Build history of the part. All positions in model axes, mm. A direction names the side the tool comes from. Round coordinates to 2 decimals unless told otherwise and drop trailing zeros. Write each loop counter-clockwise with the first axis right and the second up, starting at its lowest first coordinate (ties: lowest second). Pieces come first, ordered by that corner, then holes. Notation, with made-up numbers: (0, -38) - (15, -38) arc R28 ccw to (15, -8) - close; hole circle Ø11 at (22, -21.75). An arc over 180 degrees is marked (long way). Answer as a JSON object with one key per item and string values. Group by question number.
Item 1: Slice it at C-C, the plane z = 18. List the corners of the cut face in (x, y), then the cut area to 3 significant figures.
Item 2: Probe line 1 (Y direction, x = 7, z = 22.5); line 2 (Y direction, x = 2.5, z = -18.5); line 3 (X direction, y = 3.1, z = 18). List the from-to ranges inside material, lowest first. Write a range as from..to.
Item 3: Two-plate mould, pull along Z, no slides. Class faces 1 (the flat face through (15.586, 1.232, 1.42)), 2 (the flat face through (0, -66, -2.425)), 3 (the flat face through (0, -126, 0)): +Z half, -Z half, draft (parallel to the pull), parting line (faces both ways), or undercut.
Item 4: Slice it at A-A, the plane x = -18. List the corners of the cut face in (y, z).
Item 5: Which spindle directions (+Z, -Z, +X, -X, +Y, -Y) get a long thin tool onto all of the face, cutting with end or side? Do faces 4 (the cylindrical face through (11.538, 3.24, 13.641)), 5 (the flat face through (1.38, 1.232, -20.436)). Say none if no direction does.
Item 6: Flat gauge pins, fed straight in: pin 1 (5 mm diameter, centred on x = -12, z = -13, fed in from -Y); pin 2 (2 mm diameter, centred on x = -17.5, y = 1, fed in from -Z); pin 3 (5 mm diameter, centred on x = 0, z = 18, fed in from +Y); pin 4 (3 mm diameter, centred on y = 1, z = 19, fed in from -X). Where does each tip first touch, or does it go through?
Item 7: Slice it at B-B, the plane y = -21.5. List the corners of the cut face in (x, z) (3 decimals), then the cut area to 3 significant figures.
from build123d import *

# Parameters (mm, degrees)
SKETCH_1_R               = 20
EXTRUDE_1_DEPTH          = 4
SKETCH_2_R               = 7.407075634
EXTRUDE_2_DEPTH          = 8
SKETCH_3_W               = 4.85
SKETCH_3_H               = 4.85
EXTRUDE_3_DEPTH          = 118
SKETCH_5_R               = 25
EXTRUDE_4_DEPTH          = 4
CUT_EXTRUDE_1_DEPTH      = 2.5
SKETCH_7_R               = 1.5
CUT_EXTRUDE_2_DEPTH      = 2.5
PATTERN_CIRCULAR_1_COUNT = 8
FILLET_1_R               = 1
SKETCH_9_R               = 25
EXTRUDE_5_DEPTH          = 4
SKETCH_10_R              = 5.5
EXTRUDE_6_DEPTH          = 8
SKETCH_11_W              = 4.85
SKETCH_11_H              = 4.85
EXTRUDE_7_DEPTH          = 118
CUT_EXTRUDE_7_DEPTH      = 128.5
SKETCH_13_R              = 1.5
CUT_EXTRUDE_8_DEPTH      = 128.5
PATTERN_CIRCULAR_2_COUNT = 8
FILLET_2_R               = 1
SKETCH_14_R              = 7.407075634
SKETCH_14_R_2            = 5.5
CUT_EXTRUDE_9_DEPTH      = 8
SKETCH_15_W              = 54.152446135
SKETCH_15_H              = 58.876914062
CUT_EXTRUDE_10_DEPTH     = 130


with BuildPart() as part:
    # 草图1 → 凸台-拉伸1 (new body)
    with BuildSketch(Plane(origin=(0, 0, 0), x_dir=(1, 0, 0), z_dir=(0, 1, 0))):
        Circle(SKETCH_1_R)
    extrude(amount=EXTRUDE_1_DEPTH)

    # 草图2 → 凸台-拉伸2 (add)
    with BuildSketch(Plane.XZ):
        Circle(SKETCH_2_R)
    extrude(amount=EXTRUDE_2_DEPTH)

    # 草图3 → 凸台-拉伸3 (add)
    with BuildSketch(Plane.XZ.offset(8)):
        Rectangle(SKETCH_3_W, SKETCH_3_H)
    extrude(amount=EXTRUDE_3_DEPTH)

    # 草图5 → 凸台-拉伸4 (add)
    with BuildSketch(Plane(origin=(0, 4, 0), x_dir=(1, 0, 0), z_dir=(0, 1, 0))):
        Circle(SKETCH_5_R)
    extrude(amount=-EXTRUDE_4_DEPTH)

    # 草图6 → 切除-拉伸1 (cut)
    with BuildSketch(Plane.XZ):
        Polygon((21.233161507, 0), (19.616580754, 2.8), (16.383419246, 2.8), (14.766838493, 0), (16.383419246, -2.8), (19.616580754, -2.8), align=None)
    cut_extrude_1 = extrude(amount=-CUT_EXTRUDE_1_DEPTH, mode=Mode.SUBTRACT)

    # 草图7 → 切除-拉伸2 (cut)
    with BuildSketch(Plane.XZ.offset(-2.5)):
        with Locations((18, 0)):
            Circle(SKETCH_7_R)
    cut_extrude_2 = extrude(amount=-CUT_EXTRUDE_2_DEPTH, mode=Mode.SUBTRACT)

    # 阵列(圆周)1: 切除-拉伸1, 切除-拉伸2 ×8 about axis
    pattern_circular_1_axis = Axis((0, 0, 0), (0, 1, 0))
    for i in range(1, PATTERN_CIRCULAR_1_COUNT):
        add(cut_extrude_1.rotate(pattern_circular_1_axis, i * 360 / PATTERN_CIRCULAR_1_COUNT), mode=Mode.SUBTRACT)
        add(cut_extrude_2.rotate(pattern_circular_1_axis, i * 360 / PATTERN_CIRCULAR_1_COUNT), mode=Mode.SUBTRACT)

    # 圆角1
    fillet_1_edges = [part.edges().sort_by_distance(p)[0] for p in [
        (2.425, -67, -2.425),
        (2.425, -67, 2.425),
        (-2.425, -67, 2.425),
        (-2.425, -67, -2.425),
    ]]
    fillet(fillet_1_edges, radius=FILLET_1_R)

    # 草图14 → 切除-拉伸9 (cut)
    with BuildSketch(Plane.XZ.offset(8)):
        Circle(SKETCH_14_R)
        Circle(SKETCH_14_R_2, mode=Mode.SUBTRACT)
    extrude(amount=-CUT_EXTRUDE_9_DEPTH, mode=Mode.SUBTRACT)


with BuildPart() as body_2:
    # 草图9 → 凸台-拉伸5 (new body)
    with BuildSketch(Plane(origin=(0, 0, 0), x_dir=(1, 0, 0), z_dir=(0, 1, 0))):
        with Locations((53.487556259, 0)):
            Circle(SKETCH_9_R)
    extrude(amount=EXTRUDE_5_DEPTH)

    # 草图10 → 凸台-拉伸6 (add)
    with BuildSketch(Plane.XZ):
        with Locations((53.487556259, 0)):
            Circle(SKETCH_10_R)
    extrude(amount=EXTRUDE_6_DEPTH)

    # 草图11 → 凸台-拉伸7 (add)
    with BuildSketch(Plane.XZ.offset(8)):
        with Locations((53.487556259, 0)):
            Rectangle(SKETCH_11_W, SKETCH_11_H)
    extrude(amount=EXTRUDE_7_DEPTH)

    # 草图12 → 切除-拉伸7 (cut)
    with BuildSketch(Plane.XZ.offset(126)):
        Polygon((38.720717767, 0), (37.104137013, 2.8), (33.870975506, 2.8), (32.254394752, 0), (33.870975506, -2.8), (37.104137013, -2.8), align=None)
    cut_extrude_7 = extrude(amount=-CUT_EXTRUDE_7_DEPTH, mode=Mode.SUBTRACT)

    # 草图13 → 切除-拉伸8 (cut)
    with BuildSketch(Plane.XZ.offset(-2.5)):
        with Locations((35.487556259, 0)):
            Circle(SKETCH_13_R)
    cut_extrude_8 = extrude(amount=-CUT_EXTRUDE_8_DEPTH, mode=Mode.SUBTRACT)

    # 阵列(圆周)2: 切除-拉伸7, 切除-拉伸8 ×8 about axis
    pattern_circular_2_axis = Axis((53.487556259, 0, 0), (0, 1, 0))
    for i in range(1, PATTERN_CIRCULAR_2_COUNT):
        add(cut_extrude_7.rotate(pattern_circular_2_axis, i * 360 / PATTERN_CIRCULAR_2_COUNT), mode=Mode.SUBTRACT)
        add(cut_extrude_8.rotate(pattern_circular_2_axis, i * 360 / PATTERN_CIRCULAR_2_COUNT), mode=Mode.SUBTRACT)

    # 圆角2
    fillet_2_edges = [body_2.edges().sort_by_distance(p)[0] for p in [
        (55.912556259, -67, -2.425),
        (55.912556259, -67, 2.425),
        (51.062556259, -67, 2.425),
        (51.062556259, -67, -2.425),
    ]]
    fillet(fillet_2_edges, radius=FILLET_2_R)

    # 草图15 → 切除-拉伸10 (cut)
    with BuildSketch(Plane(origin=(0, 4, 0), x_dir=(1, 0, 0), z_dir=(0, 1, 0))):
        with Locations((53.48755626, 0)):
            Rectangle(SKETCH_15_W, SKETCH_15_H)
    extrude(amount=-CUT_EXTRUDE_10_DEPTH, mode=Mode.SUBTRACT)


solid = part.part
Geometry says:
{
 "1": {"outline": "(-17.35, 0) - (-2.8, 0) - (-2.8, 2.5) - (-1.5, 2.5) - (-1.5, 4) - (-17.35, 4) - close; (1.5, 2.5) - (2.8, 2.5) - (2.8, 0) - (17.35, 0) - (17.35, 4) - (1.5, 4) - close", "area": "120 mm^2"},
 "2": {"line 1": "y = 0..4", "line 2": "y = 2.5..4", "line 3": "x = -17.35..-1.5, 1.5..17.35"},
 "3": {"face 1": "undercut", "face 2": "-Z half", "face 3": "draft"},
 "4": {"outline": "(0, -17.35) - (4, -17.35) - (4, -1.5) - (2.5, -1.5) - (2.5, -2.8) - (0, -2.8) - close; (0, 2.8) - (2.5, 2.8) - (2.5, 1.5) - (4, 1.5) - (4, 17.35) - (0, 17.35) - close"},
 "5": {"face 4": "+Y, -Y", "face 5": "-Y"},
 "6": {"pin 1": "stops at y = 0", "pin 2": "stops at z = -18.78", "pin 3": "stops at y = 4", "pin 4": "stops at x = -17.85"},
 "7": {"outline": "(-2.425, -1.425) arc R1 ccw to (-1.425, -2.425) - (1.425, -2.425) arc R1 ccw to (2.425, -1.425) - (2.425, 1.425) arc R1 ccw to (1.425, 2.425) - (-1.425, 2.425) arc R1 ccw to (-2.425, 1.425) - close", "area": "22.7 mm^2"}
}
